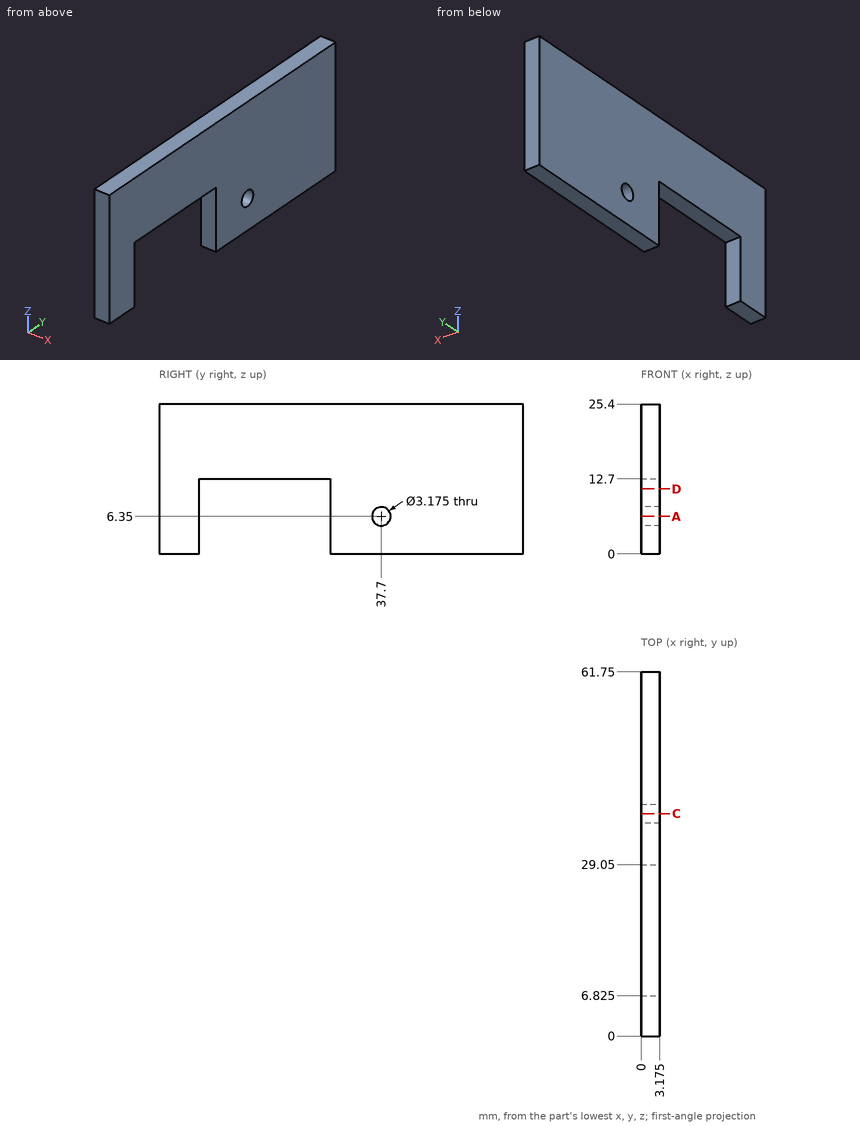
Part print with two shaded views. Sizes in mm from the minimum x, y, z corner. Round coordinates to 2 decimals unless told otherwise and drop trailing zeros. Write each loop counter-clockwise with the first axis right and the second up, starting at its lowest first coordinate (ties: lowest second). Pieces come first, ordered by that corner, then holes. Notation, with made-up numbers: M 89,67.5 L 126,67.5 A23 cw 126,81.5 Z; hole C 59,47 d5. An arc over 180 degrees is marked long. Answer as CSV lines item,"result". Start each with the question number.
1) Drop a flat-ended pin along its axis: pin 1 (1 mm diameter, centred on x = 1, y = 20, fed in from -Z). Give the stop position or say it passes through.
2) Band-saw the part on D-D (z = 11). List the corners of the cut face in (x, y) (3 decimals).
3) Band-saw the part on A-A (z = 6.35). Count the separate pieces of the cut face and the enclosed holes in it, then the cut area to 3 significant figures.
4) Band-saw the part on C-C (y = 37.7). List the corners of the cut face in (x, z) (1 decimal), then the cut area to 3 significant figures.
5) Drill centre lines: L1, parallel to Y at x = 1.95, z = 2.5 (3 decimals); L2, parallel to Z at x = 2, y = 37.7; L3, parallel to Z at x = 2.4, y = 27. Where is each one in solid material? Low to high.
Worked out:
1,pin 1,"z = 12.7"
2,outline,"M 0,0 L 3.175,0 L 3.175,6.825 L 0,6.825 Z; M 0,29.05 L 3.175,29.05 L 3.175,61.75 L 0,61.75 Z"
3,separate pieces,"3"
3,enclosed holes,"0"
3,area,"115 mm²"
4,outline,"M 0,0 L 3.2,0 L 3.2,4.8 L 0,4.8 Z; M 0,7.9 L 3.2,7.9 L 3.2,25.4 L 0,25.4 Z"
4,area,"70.6 mm²"
5,L1,"0 to 6.825, 29.05 to 61.75"
5,L2,"0 to 4.76, 7.94 to 25.4"
5,L3,"12.7 to 25.4"
